Model file for the job. Use its own axes, mm. Coordinates: 2 decimals unless noted, no trailing zeros. Order: outer loops, then holes, each group sorted by start corner. A loop starts at its lowest first (then second) coordinate and runs counter-clockwise, first axis right, second up.
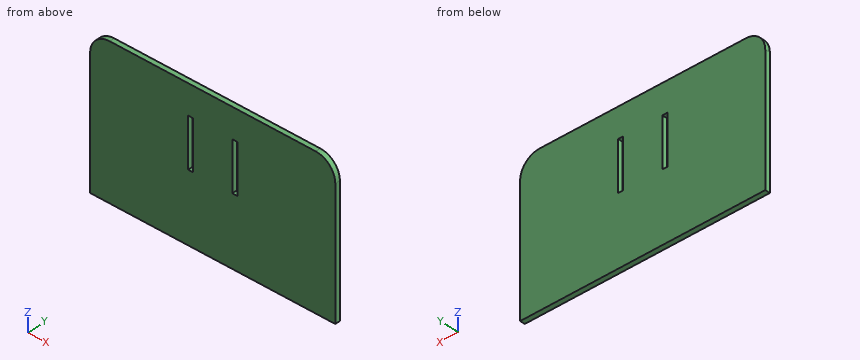
from build123d import *

# Parameters (mm, degrees)
SKETCH1_W           = 5.1
SKETCH1_H           = 50
BOSS_EXTRUDE1_DEPTH = 5.1


with BuildPart() as part:
    # Sketch1 → Boss-Extrude1 (new body)
    with BuildSketch(Plane(origin=(0, 0, 0), x_dir=(1, 0, 0), z_dir=(0, 1, 0))):
        with BuildLine():
            Line((105, -75), (-105, -75))
            ThreePointArc((-105, -75), (-119.142135624, -69.142135624), (-125, -55))
            Line((-125, -55), (-125, 75))
            Line((-125, 75), (125, 75))
            Line((125, 75), (125, -55))
            ThreePointArc((125, -55), (119.142135624, -69.142135624), (105, -75))
        make_face()
        with Locations((-22.55, -20)):
            Rectangle(SKETCH1_W, SKETCH1_H, mode=Mode.SUBTRACT)
        with Locations((22.55, -20)):
            Rectangle(SKETCH1_W, SKETCH1_H, mode=Mode.SUBTRACT)
    extrude(amount=BOSS_EXTRUDE1_DEPTH)


solid = part.part
Q1. Cut at A-A, the plane z = 19. List the corners of the cut face in (x, y).
Established:
outline: (-125, 0) - (-25.1, 0) - (-25.1, 5.1) - (-125, 5.1) - close; (-20, 0) - (20, 0) - (20, 5.1) - (-20, 5.1) - close; (25.1, 0) - (125, 0) - (125, 5.1) - (25.1, 5.1) - close
Q2. Probe line 1 (X direction, y = 4.05, z = 27); line 2 (Z direction, x = 23, y = 2.55); line 3 (Z direction, x = 109.5, y = 4.45). List the from-to ranges inside material, lowest first.
Established:
line 1: x = -125 to -25.1, -20 to 20, 25.1 to 125
line 2: z = -75 to -5, 45 to 75
line 3: z = -75 to 74.49
Q3. Cut at B-B, the plane y = 2.3. List the corners of the cut face in (x, z), plus the area to 3 significant figures.
Established:
outline: (-125, -75) - (125, -75) - (125, 55) arc R20 ccw to (105, 75) - (-105, 75) arc R20 ccw to (-125, 55) - close; hole (-25.1, -5) - (-20, -5) - (-20, 45) - (-25.1, 45) - close; hole (20, -5) - (25.1, -5) - (25.1, 45) - (20, 45) - close
area: 36,800 mm2
